Could you check a few things on this model? Use its own coordinates, in mm. Give positions to 0.01 mm unless a question says otherwise; leave off trailing zeros. Order: outer loops, then holes, each group sorted by start corner. A loop starts at its lowest first (then second) coordinate and runs counter-clockwise, first axis right, second up.
(1) If we mould it in two halves opening along Y, with no side actions, what happens to faces 1 (the cylindrical face through (-27.17, 5.29, 1.61)), 2 (the flat face through (-1, -21, 3.18))? For each: released by +Y, released by -Y, zero draft, split by the parting line, or undercut.
(2) Imagine slicing it at B-B, the plane y = 81. Write out the boundary of the cut face in (x, z), then the cut area to 3 significant figures.
(3) Imagine slicing it at C-C, the plane z = 1.3. State how many separate pieces and enclosed holes the cut face has, then the cut area to 3 significant figures.
(4) Imagine slicing it at A-A, the plane x = -18. Write out the boundary of the cut face in (y, z).
(5) Will these pins go through, and if not, where does the flat tip stop? pin 1 (1 mm diameter, centred on y = -48.5, z = 1, fed in from +X); pin 2 (1 mm diameter, centred on x = -101.5, z = 2, fed in from +Y); pin 3 (0.9 mm diameter, centred on x = 0, z = 1, fed in from +Y).
(6) If I drill on probe 1 along Y at (x, z) = (-19, 1.25); probe 2 along X at (y, z) = (4.5, 0.2); probe 3 along Y at (x, z) = (-101.43, 2), over which ranges is the centre line in solid material (lowest first)?
from build123d import *

# Parameters (mm, degrees)
SKETCH2_W           = 200
SKETCH2_H           = 200
BOSS_EXTRUDE1_DEPTH = 3.18
CUT_EXTRUDE1_DEPTH  = 142.457104452
SKETCH4_W           = 3.18
SKETCH4_H           = 10
BOSS_EXTRUDE2_DEPTH = 3.18
SKETCH6_R           = 1.47
CUT_EXTRUDE2_DEPTH  = 144.722735849
SKETCH8_W           = 40.9
SKETCH8_H           = 19.9
CUT_EXTRUDE4_DEPTH  = 144.722735849
SKETCH10_R          = 2.2225
CUT_EXTRUDE6_DEPTH  = 144.722735849


with BuildPart() as part:
    # Sketch2 → Boss-Extrude1 (new body)
    with BuildSketch(Plane.XY):
        Rectangle(SKETCH2_W, SKETCH2_H)
    extrude(amount=BOSS_EXTRUDE1_DEPTH)

    # Sketch3 → Cut-Extrude1 (cut, through all)
    with BuildSketch(Plane.XY.offset(3.18)):
        Polygon((-5, 100), (5, 100), (5, 96.82), (1.47, 96.82), (1.47, 94.74), (3.25, 94.74), (3.25, 92.14), (1.47, 92.14), (1.47, 90.07), (-1.47, 90.07), (-1.47, 92.14), (-3.25, 92.14), (-3.25, 94.74), (-1.47, 94.74), (-1.47, 96.82), (-5, 96.82), align=None)
        Polygon((1.47, -96.82), (5, -96.82), (5, -100), (-5, -100), (-5, -96.82), (-1.47, -96.82), (-1.47, -94.74), (-3.25, -94.74), (-3.25, -92.14), (-1.47, -92.14), (-1.47, -90.07), (1.47, -90.07), (1.47, -92.14), (3.25, -92.14), (3.25, -94.74), (1.47, -94.74), align=None)
    extrude(amount=-CUT_EXTRUDE1_DEPTH, mode=Mode.SUBTRACT)

    # Sketch4 → Boss-Extrude2 (add)
    with BuildSketch(Plane.ZY.offset(100)):
        with Locations((1.59, 0)):
            Rectangle(SKETCH4_W, SKETCH4_H)
    boss_extrude2 = extrude(amount=BOSS_EXTRUDE2_DEPTH)

    # Sketch6 → Cut-Extrude2 (cut, through all)
    with BuildSketch(Plane.XY.offset(3.18)):
        with Locations((-101.43, 0)):
            Circle(SKETCH6_R)
    cut_extrude2 = extrude(amount=-CUT_EXTRUDE2_DEPTH, mode=Mode.SUBTRACT)

    # Mirror1: Boss-Extrude2 across plane
    add(boss_extrude2.mirror(Plane(origin=(0, 0, 0), x_dir=(0, 0, 1), z_dir=(1, 0, 0))))

    # Mirror2: Cut-Extrude2 across plane
    add(cut_extrude2.mirror(Plane(origin=(0, 0, 0), x_dir=(0, 0, 1), z_dir=(1, 0, 0))), mode=Mode.SUBTRACT)

    # Sketch8 → Cut-Extrude4 (cut, through all)
    with BuildSketch(Plane.XY.offset(3.18)):
        Rectangle(SKETCH8_W, SKETCH8_H)
    extrude(amount=-CUT_EXTRUDE4_DEPTH, mode=Mode.SUBTRACT)

    # Sketch10 → Cut-Extrude6 (cut, through all)
    with BuildSketch(Plane.XY.offset(3.18)):
        with Locations((-24.949, 5.1875)):
            Circle(SKETCH10_R)
        with Locations((-24.949, -4.9725)):
            Circle(SKETCH10_R)
        with Locations((25.149, 5.1875)):
            Circle(SKETCH10_R)
        with Locations((25.149, -4.9725)):
            Circle(SKETCH10_R)
    extrude(amount=-CUT_EXTRUDE6_DEPTH, mode=Mode.SUBTRACT)


solid = part.part
Answer block:
1. face 1: undercut
1. face 2: zero draft
2. outline: (-100, 0) - (100, 0) - (100, 3.18) - (-100, 3.18) - close
2. area: 636 mm2
3. separate pieces: 1
3. enclosed holes: 7
3. area: 39,100 mm2
4. outline: (-100, 0) - (-9.95, 0) - (-9.95, 3.18) - (-100, 3.18) - close; (9.95, 0) - (100, 0) - (100, 3.18) - (9.95, 3.18) - close
5. pin 1: stops at x = 100
5. pin 2: stops at y = 5
5. pin 3: stops at y = 90.07
6. probe 1: y = -100 to -9.95, 9.95 to 100
6. probe 2: x = -103.18 to -27.06, -22.84 to -20.45, 20.45 to 23.04, 27.26 to 103.18
6. probe 3: y = -5 to -1.47, 1.47 to 5
